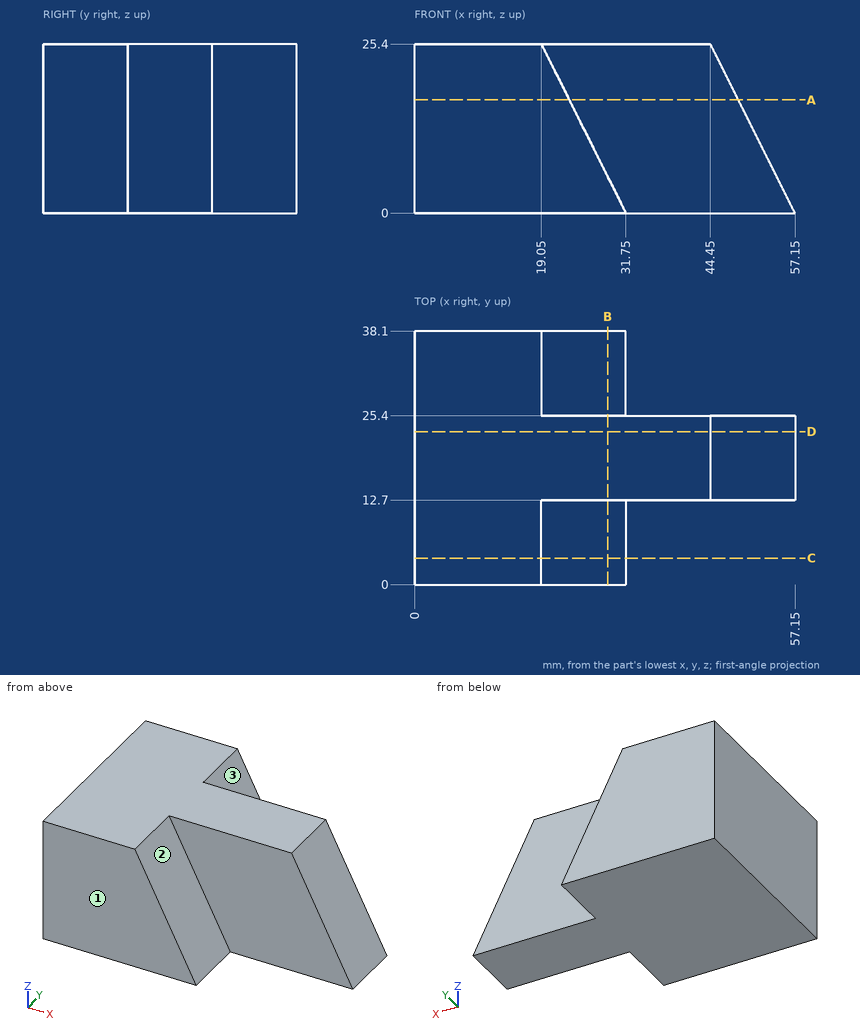
Source: three-view drawing plus pictorial views. Frame: mm from the lowest corner of the part. A direction names the side the tool comes from. Coordinates: 2 decimals unless noted, no trailing zeros. Order: outer loops, then holes, each group sorted by start corner. A loop starts at its lowest first (then second) coordinate and runs counter-clockwise, first axis right, second up. Notation, with made-up numbers: M -15,52 L 13,52 A15 ccw 13,78 Z; hole C -14.5,69 d6. An arc over 180 degrees is marked long. One line per question, with ' | ' between items. Start each with the question number.
Item 1: Cut plane C-C, the plane y = 4. Return the cut outline in (x, z), then the cut area to 3 significant figures.
Item 2: Ray query, probe 1 along Y at (x, z) = (29, 11.75); probe 2 along Z at (x, y) = (22, 7.5); probe 3 along X at (y, z) = (14, 1.25) (3 decimals). Return the intervals inside material, ascending. Write a range as [from, to].
Item 3: Set-up query: the marked faces 1, 2 and 3. Return all of +Z, -Z, +X, -X, +Y, -Y with unobstructed straight access to the full face (end or side cutting, diameter ignored); none if empty.
Item 4: Cut plane A-A, the plane z = 17. Return the cut outline in (x, y), then the cut area to 3 significant figures.
Item 5: Cut plane B-B, the plane x = 29. Return the cut outline in (y, z).
Item 6: Cut plane D-D, the plane y = 23. Return the cut outline in (x, z).
Item 7: Pin query (flat end, axial travel): pin 1 Ø3 at (x, z) = (28, 4.5) entering from -Y; pin 2 Ø5 at (x, z) = (34.5, 5) entering from +Y; pin 3 Ø2 at (y, z) = (9.5, 6) entering from +X. Return the tip coordinate at first contact, or that it passes through.
A:
1) outline: M 0,0 L 31.75,0 L 19.05,25.4 L 0,25.4 Z | area: 645 mm2
2) probe 1: y = [12.7, 25.4] | probe 2: z = [0, 19.5] | probe 3: x = [0, 56.525]
3) face 1: +Z, -Z, +X, -X, -Y | face 2: +Z, +X, -Y | face 3: +Z, +X, +Y
4) outline: M 0,0 L 23.25,0 L 23.25,12.7 L 48.65,12.7 L 48.65,25.4 L 23.25,25.4 L 23.25,38.1 L 0,38.1 Z | area: 1,210 mm2
5) outline: M 0,0 L 38.1,0 L 38.1,5.5 L 25.4,5.5 L 25.4,25.4 L 12.7,25.4 L 12.7,5.5 L 0,5.5 Z
6) outline: M 0,0 L 57.15,0 L 44.45,25.4 L 0,25.4 Z
7) pin 1: stops at y = 0 | pin 2: stops at y = 25.4 | pin 3: stops at x = 29.25
